Check sheet for the modelled part. Datum: model origin and axes. Units: mm. A direction names the side the tool comes from. Coordinates: 2 decimals unless noted, no trailing zeros. Loops run counter-clockwise (first coordinate to the right, second up) from the corner with the lowest first, then second, coordinate; pieces in that order, holes last. Notation, with made-up numbers: (50, -13.75) -> (68, -13.75) arc R16 ccw to (68, 17.25) -> close; hole circle Ø11 at (66, -27.75). An arc over 180 degrees is marked (long way). Use CSV: the item, a comma, the result in double quotes. Start each with the question number.
1. Sectioned sample at B-B, the plane x = 42. Record the cut outline in (y, z).
2. Sectioned sample at D-D, the plane z = 13.75. Record the cut outline in (x, y).
3. Gauge pin test, flat ends, axial feed: pin 1 (4 mm diameter, centred on x = 42, y = 40, fed in from -Z); pin 2 (1.5 mm diameter, centred on x = 1, z = 4.67, fed in from +Y); pin 3 (10 mm diameter, centred on x = 2, y = 43.5, fed in from +Z). Record the tip position at first contact, or that the pin passes through.
4. Sectioned sample at A-A, the plane y = 40. Record the cut outline in (x, z).
5. Release check for a two-part mould opening along Z. For faces 1 (the face through (0.631, 43.409, 5.844)), 2 (the face through (-1, 1, 0)), 3 (the face through (18.88, -3.51, 10.14)) record: pulls with the +Z half, pulls with the -Z half, needs draft (parallel to the pull), parting line crosses it, or undercut.
6. Thickness scan on L1, parallel to Y at x = 19, z = 1.75; L2, parallel to X at y = 40, z = 8.25; L3, parallel to Z at x = 1, y = 40. Record the ranges inside material, lowest first.
7. Sectioned sample at C-C, the plane y = -40. Record the cut outline in (x, z), and give its area (3 significant figures).
8. Set-up check for faces 4 (the face through (0.7, -32.927, 15.07)), 5 (the face through (-50, -1, 10)), 6 (the face through (0.7, 32.846, 14.93)): record each of +Z, -Z, +X, -X, +Y, -Y from which the full face is reachable in a straight line by a thin tool's end or side.
Autodesk Inventor part; units mm, degrees
ref_plane "YZ Plane" through (0, 0, 0) normal (1, 0, 0) x (0, 1, 0)
ref_plane "XZ Plane" through (0, 0, 0) normal (0, 1, 0) x (-1, 0, 0)
ref_plane "XY Plane" through (0, 0, 0) normal (0, 0, 1) x (1, 0, 0)
sketch "Sketch1" plane through (0, 0, 0) normal (0, 0, 1) x (1, 0, 0)
  line L0 (-50, 50) -> (50, 50)
  line L1 (50, 50) -> (50, -50)
  line L2 (50, -50) -> (-50, -50)
  line L3 (-50, -50) -> (-50, 50)
  line L4 (0, 0) -> (0, 10.7535) construction
  line L5 (0, 0) -> (8.6992, 0) construction
  dimension "d0" = 100
  dimension "d1" = 100
extrude "Extrusion1" add sketch "Sketch1" along normal blind 10
sketch "Sketch2" plane through (50, -50, 0) normal (1, 0, 0) x (0, 0, -1)
  line L0 (-10, 80) -> (-20, 85.7735)
  line L1 (-20, 85.7735) -> (-20, 14.2265)
  line L2 (-20, 14.2265) -> (-10, 20)
  line L3 (0, 0) -> (-10, 0)
  line L4 (0, 100) -> (-10, 100)
  line L5 (-10, 80) -> (-10, 20)
  line L6 (-10, 0) -> (-10, 100)
  point P0 (0, 50)
  dimension "d4" = 60
  dimension "d5" = 60
  dimension "d6" = 20
  dimension "d7" = 20
  dimension "d19" = 10
extrude "Extrusion2" add sketch "Sketch2" against normal blind 100
sketch "Sketch3" plane through (0, 0, 0) normal (0, 0, -1) x (-1, 0, 0)
  circle A0 centre (19.25, -4.6808) radius 1.6
  circle A1 centre (19.25, 25.3192) radius 1.6
  circle A2 centre (-19.25, 25.3192) radius 1.6
  circle A3 centre (-19.25, -4.6808) radius 1.6
  point P0 (0, 0)
hole "Hole1" at (19.25, 25.3192, 0) at (19.25, -4.6808, 0) at (-19.25, 25.3192, 0) at (-19.25, -4.6808, 0) direction (0, 0, 1) diameter 2.459 end through all
sketch "Sketch4" plane through (0, 0, 0) normal (0, 0, -1) x (-1, 0, 0)
  line L0 (50, -50) -> (50, 50)
  line L1 (-50, -50) -> (50, -50)
  line L2 (50, 50) -> (-50, 50)
  line L3 (-50, 50) -> (-50, -50)
  point P0 (0, 0)
  point P1 (42, -40)
  point P2 (42, 40)
  point P3 (-42, 40)
  point P4 (-42, -40)
  dimension "d20" = 8
  dimension "d21" = 10
  dimension "d22" = 10
  dimension "d23" = 8
hole "Hole2" at (-42, -40, 0) at (-42, 40, 0) at (42, 40, 0) at (42, -40, 0) direction (0, 0, 1) diameter 3.242 depth 11.8 tip angle 118
chamfer "Chamfer1" distance 0.5 angle 45 4 edges at (-42, -41.621, 0) (42, -41.621, 0) (-42, 38.379, 0) (42, 38.379, 0)
sketch "Sketch5" plane through (-50, 50, 0) normal (0, 1, 0) x (1, 0, 0)
  circle A0 centre (51, -4.6715) radius 1.6
  circle A1 centre (61, -4.6715) radius 1.6
  point P0 (50, 0)
hole "Hole3" at (1, 50, 4.6715) at (11, 50, 4.6715) direction (0, -1, 0) diameter 2.459 depth 13 tip angle 118
properties part number "3d_LM-Welding_Tooling - Upper moving base" material "Aluminium 6061-T6"
Completed:
1,outline,"(-50, 0) -> (-42.12, 0) -> (-41.62, 0.5) -> (-41.62, 10) -> (-50, 10) -> close; (-38.38, 0.5) -> (-37.88, 0) -> (37.88, 0) -> (38.38, 0.5) -> (38.38, 10) -> (30, 10) -> (35.77, 20) -> (-35.77, 20) -> (-30, 10) -> (-38.38, 10) -> close; (41.62, 0.5) -> (42.12, 0) -> (50, 0) -> (50, 10) -> (41.62, 10) -> close"
2,outline,"(-50, -32.17) -> (50, -32.17) -> (50, 32.17) -> (-50, 32.17) -> close; hole circle Ø2.46 at (-19.25, -4.68); hole circle Ø2.46 at (-19.25, 25.32); hole circle Ø2.46 at (19.25, -4.68); hole circle Ø2.46 at (19.25, 25.32)"
3,pin 1,"z = 0.12"
3,pin 2,"y = 36.71"
3,pin 3,"z = 10"
4,outline,"(-50, 0) -> (-44.12, 0) -> (-43.62, 0.5) -> (-43.62, 10) -> (-50, 10) -> close; (-40.38, 0.5) -> (-39.88, 0) -> (39.88, 0) -> (40.38, 0.5) -> (40.38, 10) -> (-40.38, 10) -> close; (43.62, 0.5) -> (44.12, 0) -> (50, 0) -> (50, 10) -> (43.62, 10) -> close; hole circle Ø2.46 at (1, 4.67); hole circle Ø2.46 at (11, 4.67)"
5,face 1,"undercut"
5,face 2,"pulls with the -Z half"
5,face 3,"needs draft"
6,L1,"-50 to -5.88, -3.48 to 24.12, 26.52 to 50"
6,L2,"-50 to -43.62, -40.38 to 40.38, 43.62 to 50"
6,L3,"0 to 3.44, 5.9 to 10"
7,outline,"(-50, 0) -> (-44.12, 0) -> (-43.62, 0.5) -> (-43.62, 10) -> (-50, 10) -> close; (-40.38, 0.5) -> (-39.88, 0) -> (39.88, 0) -> (40.38, 0.5) -> (40.38, 10) -> (-40.38, 10) -> close; (43.62, 0.5) -> (44.12, 0) -> (50, 0) -> (50, 10) -> (43.62, 10) -> close"
7,area,"935 mm²"
8,face 4,"+X, -X, -Y"
8,face 5,"+Z, -Z, -X, +Y, -Y"
8,face 6,"+X, -X, +Y"
